Model file for the job. Use its own axes, mm. A direction names the side the tool comes from. Round coordinates to 2 decimals unless told otherwise and drop trailing zeros. Loops run counter-clockwise (first coordinate to the right, second up) from the corner with the lowest first, then second, coordinate; pieces in that order, holes last. Notation, with made-up numbers: M -16.5,85.5 L 35.5,85.5 A26 cw 35.5,99.5 Z; hole C -3,-20 d9. An arc over 180 degrees is marked long. Use a Markdown table: item, result. Add a question column.
Q1. Tool access for faces 4 (the face through (140, 145, 0)), 5 (the face through (95, 2, 0)), 6 (the face through (74, 76, 5)), 7 (the face through (5, 150, 0)), 8 (the face through (112, 86.3, 0)): list every direction of +Z, -Z, +X, -X, +Y, -Y with a clear straight run to the whole face (end or side of a thin tool).
Q2. Cut at A-A (y = 68). Give the cut face in (x, z).
Q3. Cut at B-B (x = 34.5). Give the cut face in (y, z), plus the area to 3 significant figures.
Q4. Probe line 1 (X direction, y = 84.5, z = 4); line 2 (Y direction, x = 41, z = 4.5); line 3 (Y direction, x = 50, z = 1.75). List the from-to ranges inside material, lowest first. Write a range as from..to.
Q5. Pin check, flat tips, straight feed: pin 1 (3 mm diameter, centred on x = 38, z = 2.5, fed in from +Y); pin 2 (3 mm diameter, centred on x = 36.5, z = -0.5, fed in from -Y). Stop position of each tip, or through.
Q6. Cut at C-C (z = 2). Give the cut face in (x, y).
Q7. Cut at D-D (x = 75.5). Give the cut face in (y, z), plus the area to 3 significant figures.
Q8. Mould opens along X. For faces 1 (the face through (150, 74, 0)), 2 (the face through (15, 2, 0)), 3 (the face through (0, 76, 0)) say: +X half, -X half, draft (parallel to the pull), parting line (faces both ways), or undercut.
from build123d import *

# Parameters (mm, degrees)
PAD_DEPTH    = 5
SKETCH001_W  = 12.2
SKETCH001_H  = 22.6
POCKET_DEPTH = 10.001


with BuildPart() as part:
    # Sketch → Pad (new body, symmetric)
    with BuildSketch(Plane.XY):
        Polygon((150, 0), (150, 150), (140, 150), (140, 140), (10, 140), (10, 150), (0, 150), (0, 0), (15, 0), (15, 5), (55, 5), (55, 0), (95, 0), (95, 5), (135, 5), (135, 0), align=None)
    extrude(amount=PAD_DEPTH, both=True)

    # Sketch001 (on Face18 of Pad) → Pocket (cut, through all)
    with BuildSketch(Plane.XY.offset(5)):
        with Locations((37.5, 75)):
            Rectangle(SKETCH001_W, SKETCH001_H)
        with Locations((112.5, 75)):
            Rectangle(SKETCH001_W, SKETCH001_H)
    extrude(amount=-POCKET_DEPTH, mode=Mode.SUBTRACT)


solid = part.part
Checked values:
| question | item | result |
|---|---|---|
| 1 | face 4 | +Z, -Z, +Y |
| 1 | face 5 | +Z, -Z, -Y |
| 1 | face 6 | +Z, +X, -X, +Y, -Y |
| 1 | face 7 | +Z, -Z, +X, -X, +Y |
| 1 | face 8 | +Z, -Z |
| 2 | outline | M 0,-5 L 31.4,-5 L 31.4,5 L 0,5 Z; M 43.6,-5 L 106.4,-5 L 106.4,5 L 43.6,5 Z; M 118.6,-5 L 150,-5 L 150,5 L 118.6,5 Z |
| 3 | outline | M 5,-5 L 63.7,-5 L 63.7,5 L 5,5 Z; M 86.3,-5 L 140,-5 L 140,5 L 86.3,5 Z |
| 3 | area | 1,120 mm^2 |
| 4 | line 1 | x = 0..31.4, 43.6..106.4, 118.6..150 |
| 4 | line 2 | y = 5..63.7, 86.3..140 |
| 4 | line 3 | y = 5..140 |
| 5 | pin 1 | stops at y = 140 |
| 5 | pin 2 | stops at y = 5 |
| 6 | outline | M 0,0 L 15,0 L 15,5 L 55,5 L 55,0 L 95,0 L 95,5 L 135,5 L 135,0 L 150,0 L 150,150 L 140,150 L 140,140 L 10,140 L 10,150 L 0,150 Z; hole M 31.4,63.7 L 43.6,63.7 L 43.6,86.3 L 31.4,86.3 Z; hole M 106.4,63.7 L 118.6,63.7 L 118.6,86.3 L 106.4,86.3 Z |
| 7 | outline | M 0,-5 L 140,-5 L 140,5 L 0,5 Z |
| 7 | area | 1,400 mm^2 |
| 8 | face 1 | +X half |
| 8 | face 2 | undercut |
| 8 | face 3 | -X half |
